Geometry: final body of the model. Coordinates: model frame, mm. Coordinates: 2 decimals unless noted, no trailing zeros. Order: outer loops, then holes, each group sorted by start corner. A loop starts at its lowest first (then second) coordinate and runs counter-clockwise, first axis right, second up. Notation, with made-up numbers: M 23.5,48.25 L 38.5,48.25 A22 ccw 38.5,60.25 Z; hole C 16,57 d6. An arc over 180 degrees is marked long. Use CSV: the item, a comma, the result in double quotes. Start each with the question number.
1. Section query D-D on x = 8.5. Return the cut outline in (y, z).
2. Section query C-C on z = -1. Return the cut outline in (x, y).
3. Material intervals for line 1 (X direction, y = -42, z = -12.5); line 2 (Y direction, x = 12.5, z = -23); line 3 (Z direction, x = 8.5, y = -27), sorted ascending.
4. First-contact query: P1, Ø12, axis at x = 34, z = -7, coming from the +Y side; P2, Ø5, axis at y = -28.5, z = -4, coming from the +X side; P3, Ø3, axis at x = 26, z = -24.5, coming from the +Y side. Flat tips, straight axial feed; report the tip coordinate or a pass-through.
5. Section query B-B on y = -38. Return the cut outline in (x, z), and give its area (3 significant figures).
6. Pull-direction query (Z, two-part tool) for faces 1 (the cylindrical face through (12.522, -24.686, -17.188)), 2 (the flat face through (12.522, -25.425, -2.44)), 3 (the cylindrical face through (31.7, -7.9, -2.9)), 4 (the flat face through (12.522, -13.887, -18.091)); classes: pulls with the +Z half, pulls with the -Z half, needs draft (parallel to the pull), parting line crosses it, or undercut.
7. Section query A-A on z = -14. Return the cut outline in (x, y), and give its area (3 significant figures).
from build123d import *

# Parameters (mm, degrees)
F0_R     = 7.2644
F1_DEPTH = 25.4
F2_R     = 4.445
F3_DEPTH = 38.1


with BuildPart() as f1:
    # F0 (on Right) → F1 (new body)
    with BuildSketch(Plane.YZ):
        with BuildLine():
            ThreePointArc((-22.047149, -27.589325), (-19.787361, -23.752651), (-19.001454, -19.369838))
            ThreePointArc((-19.001454, -19.369838), (-24.885128, -8.701443), (-37.047349, -7.985452))
            ThreePointArc((-37.047349, -7.985452), (-41.633101, -27.035061), (-22.047149, -27.589325))
        make_face()
        with Locations((-31.615363, -19.369838)):
            Circle(F0_R, mode=Mode.SUBTRACT)
        with BuildLine():
            ThreePointArc((-37.047349, -7.985452), (-24.885128, -8.701443), (-19.001454, -19.369838))
            ThreePointArc((-19.001454, -19.369838), (-19.787361, -23.752651), (-22.047149, -27.589325))
            Line((-22.047149, -27.589325), (-5.495977, -8.322288))
            ThreePointArc((-5.495977, -8.322288), (-16.760624, -8.003509), (-14.123179, 2.952667))
            Line((-14.123179, 2.952667), (-37.047349, -7.985452))
        make_face()
        with BuildLine():
            ThreePointArc((-3.744279, -3.594939), (-7.12821, 2.540872), (-14.123179, 2.952667))
            ThreePointArc((-14.123179, 2.952667), (-16.760624, -8.003509), (-5.495977, -8.322288))
            ThreePointArc((-5.495977, -8.322288), (-4.196284, -6.115667), (-3.744279, -3.594939))
        make_face()
    extrude(amount=F1_DEPTH)

    # F2 (on Right) → F3 (join)
    with BuildSketch(Plane.YZ):
        with Locations((-12.125393, -4.282554)):
            Circle(F2_R)
    extrude(amount=F3_DEPTH)


solid = f1.part
Results list:
1,outline,"M -37.05,-7.99 A12.61 ccw long -22.05,-27.59 L -5.5,-8.32 A7.25 ccw -3.74,-3.59 A7.25 ccw -14.12,2.95 Z; hole C -31.62,-19.37 d14.53"
2,outline,"M 0,-22.41 L 25.4,-22.41 L 25.4,-15.12 L 38.1,-15.12 L 38.1,-9.13 L 25.4,-9.13 L 25.4,-4.22 L 0,-4.22 Z"
3,line 1,"x = 0 to 25.4"
3,line 2,"y = -43.7 to -37.91, -25.32 to -18.1"
3,line 3,"z = -31.11 to -24.98, -13.76 to -3.19"
4,P1,"stops at y = -7.68"
4,P2,"stops at x = 25.4"
4,P3,"stops at y = -18.21"
5,outline,"M 0,-30.25 L 25.4,-30.25 L 25.4,-22.84 L 0,-22.84 Z; M 0,-15.9 L 25.4,-15.9 L 25.4,-8.49 L 0,-8.49 Z"
5,area,"377 mm²"
6,face 1,"undercut"
6,face 2,"pulls with the +Z half"
6,face 3,"parting line crosses it"
6,face 4,"pulls with the -Z half"
7,outline,"M 0,-43.03 L 25.4,-43.03 L 25.4,-36.51 L 0,-36.51 Z; M 0,-26.72 L 25.4,-26.72 L 25.4,-10.37 L 0,-10.37 Z"
7,area,"581 mm²"
